The figure shows three views and two pictorial views of one solid part (mm, origin at its lowest corner). Answer the questions. Round coordinates to 2 decimals unless told otherwise and drop trailing zeros. Order: outer loops, then holes, each group sorted by start corner. A loop starts at its lowest first (then second) coordinate and runs counter-clockwise, first axis right, second up. Notation, with made-up numbers: (75.25, 18.5) -> (96.25, 18.5) arc R30 cw to (96.25, 46.5) -> close; hole circle Ø3 at (35, -10.75). An arc over 180 degrees is marked (long way). One line per item, written item: value. Start each with the question number.
1. Section C-C (x = 4.41) is taken. Give the vertices of the cut face in (y, z) (3 decimals), then the cut area to 3 significant figures.
2. Section D-D (y = 17) is taken. Give the vertices of the cut face in (x, z) (3 decimals), then the cut area to 3 significant figures.
3. A flat-ended cylindrical pin translates along its axis: pin 1 Ø2 at (x, y) = (20.41, 17) entering from +Z. Find the tip coordinate at first contact, or state that the pin passes through.
4. Section B-B (z = 0.6) is taken. Give the vertices of the cut face in (x, y) (3 decimals).
5. Consider line 1 (X direction, y = 32, z = 2.25); line 2 (X direction, y = 3.5, z = 3.55); line 3 (Y direction, x = 22, z = 5.45). Determine where each line is inside the solid, lowest interval first.
6. Section A-A (y = 3) is taken. Give the vertices of the cut face in (x, z).
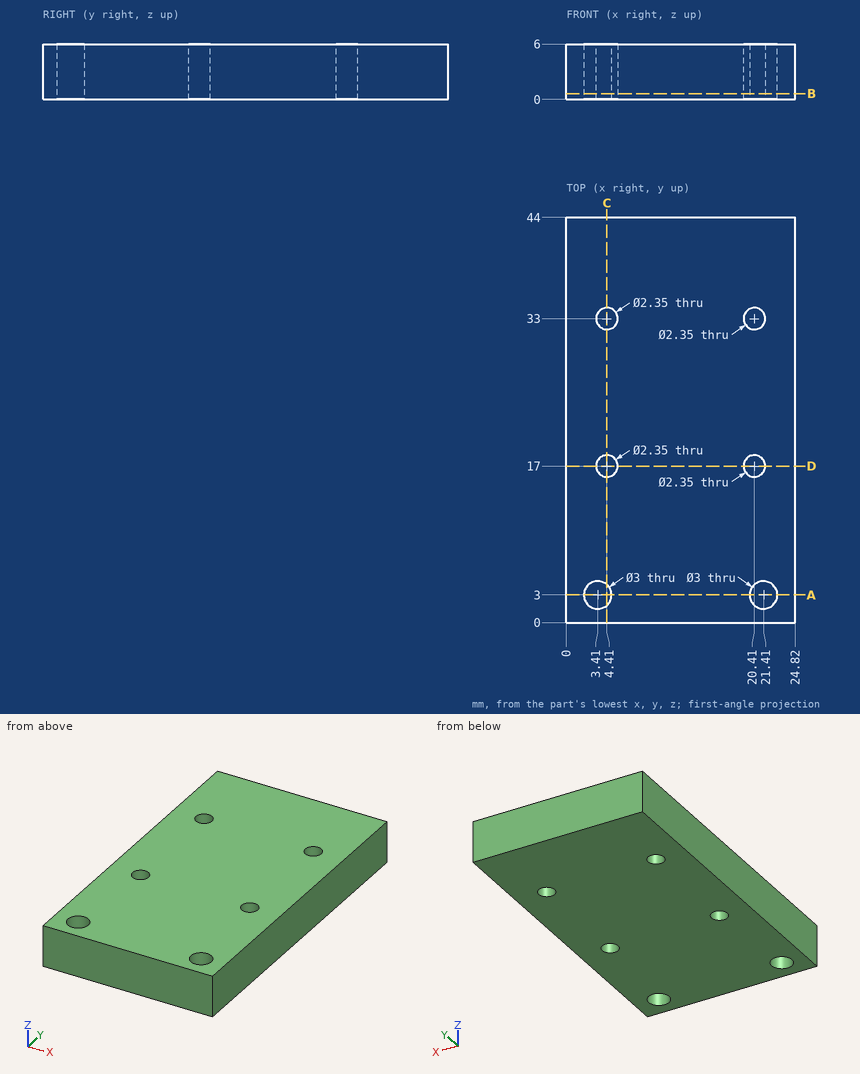
Answer:
1. outline: (0, 0) -> (1.882, 0) -> (1.882, 6) -> (0, 6) -> close; (4.118, 0) -> (15.825, 0) -> (15.825, 6) -> (4.118, 6) -> close; (18.175, 0) -> (31.825, 0) -> (31.825, 6) -> (18.175, 6) -> close; (34.175, 0) -> (44, 0) -> (44, 6) -> (34.175, 6) -> close
1. area: 222 mm^2
2. outline: (0, 0) -> (3.235, 0) -> (3.235, 6) -> (0, 6) -> close; (5.585, 0) -> (19.235, 0) -> (19.235, 6) -> (5.585, 6) -> close; (21.585, 0) -> (24.82, 0) -> (24.82, 6) -> (21.585, 6) -> close
2. area: 121 mm^2
3. pin 1: through
4. outline: (0, 0) -> (24.82, 0) -> (24.82, 44) -> (0, 44) -> close; hole circle Ø3 at (3.41, 3); hole circle Ø2.35 at (4.41, 17); hole circle Ø2.35 at (4.41, 33); hole circle Ø2.35 at (20.41, 17); hole circle Ø2.35 at (20.41, 33); hole circle Ø3 at (21.41, 3)
5. line 1: 0 to 3.79, 5.03 to 19.79, 21.03 to 24.82
5. line 2: 0 to 2, 4.82 to 20, 22.82 to 24.82
5. line 3: 0 to 1.62, 4.38 to 44
6. outline: (0, 0) -> (1.91, 0) -> (1.91, 6) -> (0, 6) -> close; (4.91, 0) -> (19.91, 0) -> (19.91, 6) -> (4.91, 6) -> close; (22.91, 0) -> (24.82, 0) -> (24.82, 6) -> (22.91, 6) -> close
